The drawing under review shows one solid part. Ordinate dimensions are in mm from its lowest x, y, z. Coordinates: 2 decimals unless noted, no trailing zeros. Loops run counter-clockwise (first coordinate to the right, second up) from the corner with the lowest first, then second, coordinate; pieces in that order, holes last. Notation, with made-up numbers: M 14.5,40 L 67.5,40 A35 cw 67.5,78 Z; hole C -36,8.25 d10. An arc over 180 degrees is marked long. Use one line per item in the form item = value.
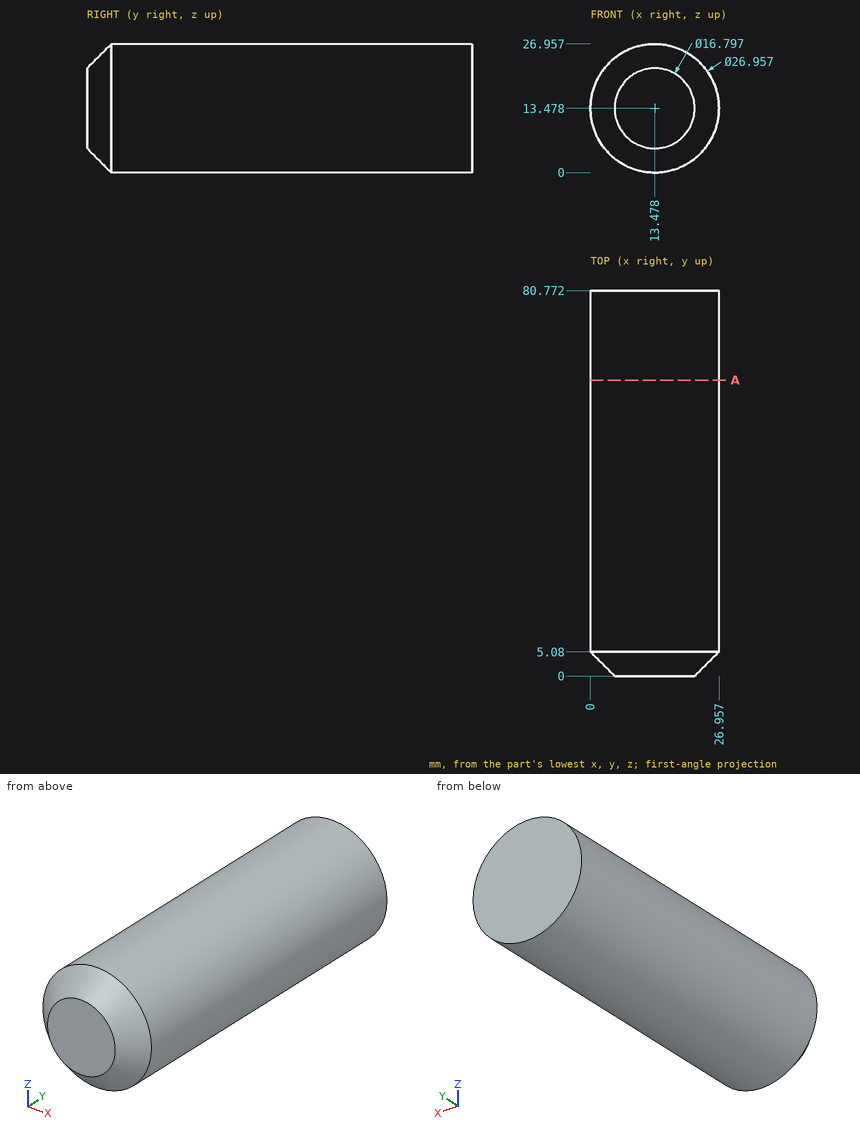
1. Consider section A-A on y = 62. Write out the cut boundary in (x, z).
Computed values:
outline = C 13.48,13.48 d26.96
2. Wall thickness on line 1 along X through (y, z) = (36, 14.25) (1 decimal); line 2 along Z through (x, y) = (6.5, 17.5); line 3 along Y through (x, z) = (5.75, 9.25): over which ranges is each line inside the solid? List them lowest first. Write a range as from..to.
Computed values:
line_1 = 0..26.9
line_2 = 1.95..25.01
line_3 = 0.41..80.77
3. For pin 1 Ø6 at (x, y) = (10, 57.5) entering from -Z; pin 2 Ø2 at (y, z) = (12, 10.5) entering from +X; pin 3 Ø1.5 at (x, y) = (19, 19) entering from +Z, all flat-tipped, find the tip position at first contact; note any pin that passes through.
Computed values:
pin_1 = 0.01
pin_2 = 26.81
pin_3 = 26.08
